Geometry: final body of the model. Coordinates: model frame, mm. A direction names the side the tool comes from. Give positions to 0.01 mm unless a question says otherwise; leave off trailing zeros. Write each loop counter-clockwise with the first axis right and the second up, starting at its lowest first coordinate (ties: lowest second). Pieces come first, ordered by that corner, then holes.
Q1. Cut plane C-C on z = -11.75. Return the cut outline in (x, y).
Q2. Pin query (flat end, axial travel): pin 1 (5.5 mm diameter, centred on y = 8.5, z = -18, fed in from +X); pin 2 (2.5 mm diameter, centred on x = 9.5, z = -12, fed in from -Y); pin 3 (2.5 mm diameter, centred on x = 12, z = -8, fed in from +Y). Return the tip coordinate at first contact, or that it passes through.
Q3. Cut plane B-B on y = -12. Return the cut outline in (x, z).
Q4. Line query: L1, parallel to Z at x = -11.5, y = -6; L2, parallel to Y at x = -7, z = -2.25; L3, parallel to X at y = -13.25, z = -4. Output: solid intervals per line, ascending.
Q5. Cut plane D-D on x = 8.25. Return the cut outline in (y, z).
Q6. Cut plane A-A on x = 2.75. Return the cut outline in (y, z).
Q7. Reachability of faces 1 (the face through (-0.8, -10, -2)), 2 (the face through (-2, 10, -15)), 3 (the face through (10, -0.8, -7)), 4 (the face through (-5, -10, -7)) from +Z, -Z, +X, -X, +Y, -Y: full face, straight path, thin tool, end or side. Return the list, or none.
Autodesk Inventor part; units mm, degrees
ref_plane "YZ Plane" through (0, 0, 0) normal (1, 0, 0) x (0, 1, 0)
ref_plane "XZ Plane" through (0, 0, 0) normal (0, 1, 0) x (-1, 0, 0)
ref_plane "XY Plane" through (0, 0, 0) normal (0, 0, 1) x (1, 0, 0)
sketch "草圖15" plane through (0, 0, 0) normal (0, 0, 1) x (1, 0, 0)
  line L0 (5, -5) -> (-5, -5)
  line L1 (-5, -5) -> (-5, 5)
  line L2 (-5, 5) -> (5, 5)
  line L3 (5, 5) -> (5, -5)
  line L4 (5, -5) -> (-5, 5) construction
  line L5 (-5, -5) -> (5, 5) construction
  line L6 (15, -15) -> (-15, -15)
  line L7 (-15, -15) -> (-15, 15)
  line L8 (-15, 15) -> (15, 15)
  line L9 (15, 15) -> (15, -15)
  line L10 (15, -15) -> (-15, 15) construction
  line L11 (-15, -15) -> (15, 15) construction
  line L12 (-15, -15) -> (-0.8, -15)
  line L13 (-0.8, -15) -> (-0.8, -5)
  line L14 (-0.8, -5) -> (-15, -5)
  line L15 (-15, -5) -> (-15, -15)
  line L16 (15, -15) -> (-1.6, -15)
  line L17 (-1.6, -5) -> (15, -5)
  line L18 (15, -5) -> (15, -15)
  line L19 (15, -15) -> (5, -15)
  line L20 (5, -15) -> (5, -0.8)
  line L21 (5, -0.8) -> (15, -0.8)
  line L22 (15, -0.8) -> (15, -15)
  line L23 (15, 15) -> (5, 15)
  line L24 (5, 15) -> (5, -1.6)
  line L25 (15, -1.6) -> (15, 15)
  line L26 (15, 15) -> (0.8, 15)
  line L27 (0.8, 15) -> (0.8, 5)
  line L28 (0.8, 5) -> (15, 5)
  line L29 (15, 5) -> (15, 15)
  line L30 (-15, 15) -> (1.6, 15)
  line L31 (1.6, 5) -> (-15, 5)
  line L32 (-15, 5) -> (-15, 15)
  line L33 (-5, -5) -> (-15, -5)
  line L34 (-15, -5) -> (-15, -15)
  line L35 (-15, -15) -> (-5, -15)
  line L36 (-5, -15) -> (-5, -5)
  line L37 (-0.8, -15) -> (-6.6, -15)
  line L38 (-6.6, -15) -> (-6.6, -5)
  line L39 (-6.6, -5) -> (-0.8, -5)
  line L40 (-0.8, -5) -> (-0.8, -15)
  line L41 (5, -0.8) -> (15, -0.8)
  line L42 (15, -0.8) -> (15, -6.6)
  line L43 (15, -6.6) -> (5, -6.6)
  line L44 (5, -6.6) -> (5, -0.8)
  line L45 (0.8, 5) -> (6.6, 5)
  line L46 (6.6, 5) -> (6.6, 15)
  line L47 (6.6, 15) -> (0.8, 15)
  line L48 (0.8, 15) -> (0.8, 5)
  line L49 (0.8, 5) -> (-5, 5)
  line L50 (-5, 5) -> (-5, 15)
  line L51 (-5, 15) -> (0.8, 15)
  line L52 (0.8, 15) -> (0.8, 5)
  point P0 (0, 0)
  point P1 (0, 0)
  point P2 (-15, -5)
  point P3 (15, -0.8)
  point P4 (5, -15)
  point P5 (0.8, 15)
  point P6 (-15, 5)
  point P7 (-5, 5)
  point P8 (15, -5)
  point P9 (-5, -15)
  point P10 (5, 5)
  point P11 (5, 15)
  point P12 (0.8, 15)
  point P13 (-6.6, -5)
  point P14 (-6.6, -15)
  point P15 (5, -6.6)
  point P16 (15, -6.6)
  point P17 (-5, 5)
  point P18 (5, 5)
  point P19 (6.6, 5)
  point P20 (6.6, 15)
  dimension "d38" = 10
  dimension "d39" = 10
  dimension "d40" = 0.8
  dimension "d42" = 0.8
  dimension "d48" = 0.8
  dimension "d54" = 0
  dimension "d55" = 5.8
  dimension "d56" = 5.8
  dimension "d57" = 5.8
  dimension "d58" = 10
extrude "擠出10" add sketch "草圖15" against normal blind 5 contours L13 L6 L36 L0 | L36 L6 L38 L14 | L38 L6 L7 L14
extrude "擠出11" add sketch "草圖15" against normal blind 5 from surface at -5 contours L20 L6 L13 L0 | L3 L21 L9 L17 | L17 L9 L43 L20 | L13 L6 L36 L0 | L43 L9 L6 L20
extrude "擠出12" add sketch "草圖15" against normal blind 5 from surface at -10 contours L3 L21 L9 L17 | L17 L9 L43 L20 | L3 L28 L9 L21 | L2 L27 L8 L24 | L24 L8 L46 L28 | L46 L8 L9 L28
extrude "擠出13" add sketch "草圖15" against normal blind 5 from surface at -15 contours L2 L27 L8 L24 | L24 L8 L46 L28 | L50 L8 L27 L2
equation "\"d39\" = width"
equation "\"d55\" = stack"
equation "\"d56\" = stack"
equation "\"d57\" = stack"
equation "\"d44\" = height"
equation "\"d46\" = height"
equation "\"d50\" = height"
equation "\"d52\" = height"
equation "\"width\" = 10"
equation "\"height\" = 5"
equation "\"gap\" = 0.8"
equation "\"stack\" = 5.8"
properties part number "Template_ladder_2"
Data:
1. outline: (0.8, 5) - (5, 5) - (5, -6.6) - (15, -6.6) - (15, 15) - (0.8, 15) - close
2. pin 1: stops at x = 6.6
2. pin 2: stops at y = -6.6
2. pin 3: stops at y = -0.8
3. outline: (-15, -5) - (-5, -5) - (-5, -10) - (15, -10) - (15, -5) - (-0.8, -5) - (-0.8, 0) - (-15, 0) - close
4. L1: z = -5 to 0
4. L2: y = -15 to -5
4. L3: x = -15 to -0.8
5. outline: (-15, -10) - (-6.6, -10) - (-6.6, -15) - (15, -15) - (15, -10) - (-0.8, -10) - (-0.8, -5) - (-15, -5) - close
6. outline: (-15, -10) - (-5, -10) - (-5, -5) - (-15, -5) - close; (5, -20) - (15, -20) - (15, -10) - (5, -10) - close
7. face 1: +Z, +X, +Y, -Y
7. face 2: +Z, -X, +Y, -Y
7. face 3: +Z, +X, -X, +Y
7. face 4: -Z, -X, +Y, -Y
